Autodesk Fusion 360 part; units mm, degrees
sketch "Plate" plane through (0, 0, 0) normal (0, 0, 1) x (1, 0, 0)
  line L0 (-111, 0.4) -> (111, 0.4)
  line L1 (111, 0.4) -> (111, 44.05)
  line L2 (111, 44.05) -> (-111, 44.05)
  line L3 (-111, 44.05) -> (-111, 0.4)
extrude "Plate (1)" add sketch "Plate" along normal blind 4
sketch "Duct walls" plane through (0, 0, 0) normal (0, 0, 1) x (1, 0, 0)
  line L0 (-97.22, 2.1) -> (97.22, 2.1)
  line L1 (97.22, 2.1) -> (97.22, 4.3)
  line L2 (97.22, 4.3) -> (-97.22, 4.3)
  line L3 (-97.22, 4.3) -> (-97.22, 2.1)
  line L4 (-97.22, 40.15) -> (97.22, 40.15)
  line L5 (97.22, 40.15) -> (97.22, 42.35)
  line L6 (97.22, 42.35) -> (-97.22, 42.35)
  line L7 (-97.22, 42.35) -> (-97.22, 40.15)
extrude "Duct walls (1)" add sketch "Duct walls" against normal blind 72
sketch "Openings and holes" plane through (0, 0, 0) normal (0, 0, 1) x (1, 0, 0)
  circle A0 centre (-63.55, 22.225) radius 19.5
  circle A1 centre (-79.55, 6.225) radius 1.8
  circle A2 centre (-79.55, 38.225) radius 1.8
  circle A3 centre (-47.55, 6.225) radius 1.8
  circle A4 centre (-47.55, 38.225) radius 1.8
  circle A5 centre (0, 22.225) radius 19.5
  circle A6 centre (-16, 6.225) radius 1.8
  circle A7 centre (-16, 38.225) radius 1.8
  circle A8 centre (16, 6.225) radius 1.8
  circle A9 centre (16, 38.225) radius 1.8
  circle A10 centre (63.55, 22.225) radius 19.5
  circle A11 centre (47.55, 6.225) radius 1.8
  circle A12 centre (47.55, 38.225) radius 1.8
  circle A13 centre (79.55, 6.225) radius 1.8
  circle A14 centre (79.55, 38.225) radius 1.8
  circle A15 centre (-102.82, 15) radius 1.7
  circle A16 centre (-102.82, 29.45) radius 1.7
  circle A17 centre (102.82, 15) radius 1.7
  circle A18 centre (102.82, 29.45) radius 1.7
extrude "Openings and holes (1)" cut sketch "Openings and holes" along normal blind 4
sketch "Tie slots" plane through (0, 0, 0) normal (0, 0, 1) x (1, 0, 0)
  line L0 (-90.69, 15) -> (-88.19, 15)
  line L1 (-88.19, 15) -> (-88.19, 20)
  line L2 (-88.19, 20) -> (-90.69, 20)
  line L3 (-90.69, 20) -> (-90.69, 15)
  line L4 (-90.69, 24.5) -> (-88.19, 24.5)
  line L5 (-88.19, 24.5) -> (-88.19, 29.5)
  line L6 (-88.19, 29.5) -> (-90.69, 29.5)
  line L7 (-90.69, 29.5) -> (-90.69, 24.5)
  line L8 (-33.03, 15) -> (-30.53, 15)
  line L9 (-30.53, 15) -> (-30.53, 20)
  line L10 (-30.53, 20) -> (-33.03, 20)
  line L11 (-33.03, 20) -> (-33.03, 15)
  line L12 (-33.03, 24.5) -> (-30.53, 24.5)
  line L13 (-30.53, 24.5) -> (-30.53, 29.5)
  line L14 (-30.53, 29.5) -> (-33.03, 29.5)
  line L15 (-33.03, 29.5) -> (-33.03, 24.5)
  line L16 (30.53, 15) -> (33.03, 15)
  line L17 (33.03, 15) -> (33.03, 20)
  line L18 (33.03, 20) -> (30.53, 20)
  line L19 (30.53, 20) -> (30.53, 15)
  line L20 (30.53, 24.5) -> (33.03, 24.5)
  line L21 (33.03, 24.5) -> (33.03, 29.5)
  line L22 (33.03, 29.5) -> (30.53, 29.5)
  line L23 (30.53, 29.5) -> (30.53, 24.5)
  line L24 (88.19, 15) -> (90.69, 15)
  line L25 (90.69, 15) -> (90.69, 20)
  line L26 (90.69, 20) -> (88.19, 20)
  line L27 (88.19, 20) -> (88.19, 15)
  line L28 (88.19, 24.5) -> (90.69, 24.5)
  line L29 (90.69, 24.5) -> (90.69, 29.5)
  line L30 (90.69, 29.5) -> (88.19, 29.5)
  line L31 (88.19, 29.5) -> (88.19, 24.5)
extrude "Tie slots (1)" cut sketch "Tie slots" along normal blind 4
ref_plane "WorkPlane1" through (0, 0, 4) normal (0, 0, 1) x (1, 0, 0)
sketch "Head counterbores" plane through (0, 0, 4) normal (0, 0, 1) x (1, 0, 0)
  circle A0 centre (-102.82, 15) radius 3.25
  circle A1 centre (-102.82, 29.45) radius 3.25
  circle A2 centre (102.82, 15) radius 3.25
  circle A3 centre (102.82, 29.45) radius 3.25
extrude "Head counterbores (1)" cut sketch "Head counterbores" against normal blind 2
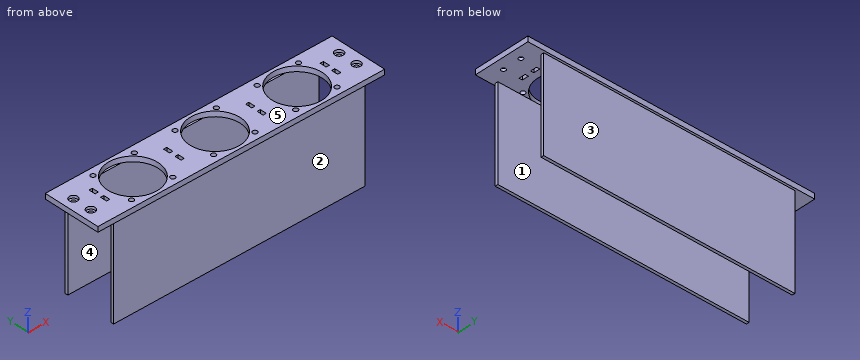
Can you work these out from the model? Positions are in its coordinate system, mm. Face numbers are marked on the shaded views. A direction names the side the tool comes from. Give positions to 0.01 mm unless a question says otherwise; leave off trailing zeros. Loops run counter-clockwise (first coordinate to the right, second up) from the corner with the lowest first, then second, coordinate; pieces in that order, holes last. Notation, with made-up numbers: M 51,-20.75 L 64,-20.75 A20 ccw 64,-0.75 Z; hole C 88,32.5 d2. An arc over 180 degrees is marked long. Use CSV: the item, a comma, the result in double quotes. Start each with the question number.
1. On a 3-axis mill with a long thin cutter (end or side, diameter ignored), from which of +Z, -Z, +X, -X, +Y, -Y can I reach the whole of each face in a straight line? I mean the marked faces 1, 2 and 3. Say none if no direction works.
2. Imagine slicing it at C-C, the plane x = -39. Write out the boundary of the cut face in (y, z).
3. If I drill on L1, parallel to Y at x = -102.82, z = 1.2; L2, parallel to Y at x = 63.55, z = 0.8 (3 decimals); L3, parallel to Y at x = -3, z = -20, over which ranges is the centre line in solid material (lowest first)?
4. Imagine slicing it at B-B, the plane z = -36. Write out the boundary of the cut face in (x, y), plus the area to 3 significant figures.
5. Imagine slicing it at A-A, the plane x = 0. Write out the boundary of the cut face in (y, z) (3 decimals), plus the area to 3 significant figures.
6. If we mould it in two halves opening along Z, with no side actions, what happens to the marked faces 4 and 5? For each: released by +Z, released by -Z, zero draft, split by the parting line, or undercut.
7. For P1, Ø4.5, axis at x = 102.82, y = 15, coming from the +Z side; P2, Ø1.5, axis at y = 6.5, z = -53, coming from the -X side; P3, Ø4, axis at x = -13, z = -40.5, coming from the +Y side; P4, Ø5, axis at y = 6.5, z = -21.5, coming from the -X side, each with a flat end and sliding along its axis, tell me the tip position at first contact or that it passes through.
Response values:
1,face 1,"-Z, +X, -X"
1,face 2,"-Z, +X, -X, -Y"
1,face 3,"-Z, +X, -X, +Y"
2,outline,"M 0.4,0 L 2.1,0 L 2.1,-72 L 4.3,-72 L 4.3,0 L 40.15,0 L 40.15,-72 L 42.35,-72 L 42.35,0 L 44.05,0 L 44.05,4 L 0.4,4 Z"
3,L1,"0.4 to 13.3, 16.7 to 27.75, 31.15 to 44.05"
3,L2,"0.4 to 2.725, 41.725 to 44.05"
3,L3,"2.1 to 4.3, 40.15 to 42.35"
4,outline,"M -97.22,2.1 L 97.22,2.1 L 97.22,4.3 L -97.22,4.3 Z; M -97.22,40.15 L 97.22,40.15 L 97.22,42.35 L -97.22,42.35 Z"
4,area,"856 mm^2"
5,outline,"M 0.4,0 L 2.1,0 L 2.1,-72 L 4.3,-72 L 4.3,0 L 2.725,0 L 2.725,4 L 0.4,4 Z; M 40.15,-72 L 42.35,-72 L 42.35,0 L 44.05,0 L 44.05,4 L 41.725,4 L 41.725,0 L 40.15,0 Z"
5,area,"335 mm^2"
6,face 4,"zero draft"
6,face 5,"released by +Z"
7,P1,"z = 2"
7,P2,"through"
7,P3,"y = 42.35"
7,P4,"x = -97.22"
